Part model, mm, in its own coordinate system. A direction names the side the tool comes from. Coordinates: 2 decimals unless noted, no trailing zeros. Loops run counter-clockwise (first coordinate to the right, second up) from the corner with the lowest first, then second, coordinate; pieces in that order, holes last.
```python
from build123d import *

# Parameters (mm, degrees)
BOSS_EXTRUDE1_DEPTH     = 40
CUT_EXTRUDE1_DEPTH      = 2
CUT_EXTRUDE1_DEPTH_BACK = 34
SKETCH5_R               = 7.241016292
CUT_EXTRUDE2_DEPTH      = 19
SKETCH4_W               = 56.944481184
SKETCH4_H               = 24.913210518
SKETCH4_W_2             = 92.534781926
SKETCH4_H_2             = 83.281303733
CUT_EXTRUDE3_DEPTH      = 19
FILLET1_R               = 10
FILLET2_R               = 10
FILLET5_R               = 20
FILLET6_R               = 20
FILLET11_R              = 10
FILLET12_R              = 10


with BuildPart() as part:
    # Sketch1 → Boss-Extrude1 (new body)
    with BuildSketch(Plane.XY):
        Polygon((-15.339960816, 87.909775446), (15.339960816, 87.909775446), (96.75975284, 65.883165043), (99.51307914, 15.143294652), (65.29316655, -26.549932182), (65.29316655, -87.909775446), (-65.29316655, -87.909775446), (-65.29316655, -26.549932182), (-99.51307914, 15.143294652), (-96.75975284, 65.883165043), align=None)
    extrude(amount=BOSS_EXTRUDE1_DEPTH)

    # Sketch3 → Cut-Extrude1 (cut, two sides: drawn at the far end of the back side and taken through both)
    with BuildSketch(Plane.XY.offset(40).offset(-CUT_EXTRUDE1_DEPTH_BACK)):
        Polygon((-92.534781925, 62.816880807), (-16.371538341, 83.815158244), (15.303829318, 83.815158244), (92.673798797, 62.816880807), (95.770608339, 16.193586837), (62.268759659, -24.735259015), (62.268759659, -84.882867266), (60.147608251, -84.882867266), (-61.571220281, -84.882867266), (-61.571220281, -24.735259015), (-95.026102977, 16.193586837), align=None)
    extrude(amount=CUT_EXTRUDE1_DEPTH + CUT_EXTRUDE1_DEPTH_BACK, mode=Mode.SUBTRACT)

    # Sketch5 → Cut-Extrude2 (cut)
    with BuildSketch(Plane(origin=(0, 87.909775446, 0), x_dir=(1, 0, 0), z_dir=(0, 1, 0))):
        with Locations(Location((0, -19.844342197, 0), (0, 0, 270))):
            Circle(SKETCH5_R)
    extrude(amount=-CUT_EXTRUDE2_DEPTH, mode=Mode.SUBTRACT)

    # Sketch4 → Cut-Extrude3 (cut)
    with BuildSketch(Plane.XY.offset(6)):
        with Locations((0, 44.665827429)):
            Rectangle(SKETCH4_W, SKETCH4_H)
        with Locations((0, -35.05644623)):
            Rectangle(SKETCH4_W_2, SKETCH4_H_2)
    extrude(amount=-CUT_EXTRUDE3_DEPTH, mode=Mode.SUBTRACT)

    # Fillet1
    fillet1_edges = [part.edges().sort_by_distance(p)[0] for p in [
        (96.75975284, 65.883165043, 20),
    ]]
    fillet(fillet1_edges, radius=FILLET1_R)

    # Fillet2
    fillet2_edges = [part.edges().sort_by_distance(p)[0] for p in [
        (-96.75975284, 65.883165043, 20),
    ]]
    fillet(fillet2_edges, radius=FILLET2_R)

    # Fillet5
    fillet5_edges = [part.edges().sort_by_distance(p)[0] for p in [
        (-99.51307914, 15.143294652, 20),
    ]]
    fillet(fillet5_edges, radius=FILLET5_R)

    # Fillet6
    fillet6_edges = [part.edges().sort_by_distance(p)[0] for p in [
        (99.51307914, 15.143294652, 20),
    ]]
    fillet(fillet6_edges, radius=FILLET6_R)

    # Fillet11
    fillet11_edges = [part.edges().sort_by_distance(p)[0] for p in [
        (65.29316655, -87.909775446, 20),
    ]]
    fillet(fillet11_edges, radius=FILLET11_R)

    # Fillet12
    fillet12_edges = [part.edges().sort_by_distance(p)[0] for p in [
        (-65.29316655, -87.909775446, 20),
    ]]
    fillet(fillet12_edges, radius=FILLET12_R)


solid = part.part
```
Q1. Probe line 1 (X direction, y = -36, z = 9); line 2 (Y direction, x = 13.5, z = 6.5); line 3 (Y direction, x = -38.5, z = 27.5). List the from-to ranges inside material, lowest first.
Q2. Mould opens along Z. For faces 5 (the flat face through (0, 85, 40)), 6 (the flat face through (-93.798, 39.179, 22.762)), 7 (the cylindrical face through (-4.41, 85.89, 14.1)) say: released by +Z, released by -Z, zero draft, split by the parting line, or undercut.
Q3. Saw through at C-C (z = 30.5). List the corners of the cut face in (x, y).
Q4. Saw through at B-B (y = -55). List the corners of the cut face in (x, z).
Q5. Drop flat-ended pins along their axis: P1, Ø5, axis at y = -31.5, z = 3.5, coming from the -X side; P2, Ø2, axis at x = 27.5, z = 8, coming from the +Y side; P3, Ø16.5, axis at x = 0, z = 19.84, coming from the +Y side; P4, Ø5, axis at y = -41, z = 8.5, coming from the +X side. Give the stop position or say it passes through.
Q6. Saw through at A-A (x = 0). List the corners of the cut face in (y, z), plus the area to 3 significant figures.
Q7. Tool access for faces 1 (the flat face through (62.269, -54, 23)), 2 (the flat face through (65.293, -52, 20)), 3 (the flat face through (-65.293, -53, 20)), 4 (the flat face through (0, 57.122, 3)): list every direction of +Z, -Z, +X, -X, +Y, -Y with a clear straight run to the whole face (end or side of a thin tool).
Q8. Saw through at D-D (y = -18.5). List the corners of the cut face in (x, z).
Checked values:
1. line 1: x = -65.29 to -61.57, 62.27 to 65.29
1. line 2: y = -87.91 to -84.88, 83.82 to 87.91
1. line 3: y = -87.91 to -84.88, 77.71 to 81.64
2. face 5: released by +Z
2. face 6: zero draft
2. face 7: undercut
3. outline: (-99.09, 22.91) arc R20 ccw to (-94.58, 9.13) - (-65.29, -26.55) - (-65.29, -77.91) arc R10 ccw to (-55.29, -87.91) - (55.29, -87.91) arc R10 ccw to (65.29, -77.91) - (65.29, -26.55) - (94.58, 9.13) arc R20 ccw to (99.09, 22.91) - (97.15, 58.66) arc R10 ccw to (89.78, 67.77) - (15.34, 87.91) - (-15.34, 87.91) - (-89.78, 67.77) arc R10 ccw to (-97.15, 58.66) - close; hole (-95.03, 16.19) - (-61.57, -24.74) - (-61.57, -84.88) - (62.27, -84.88) - (62.27, -24.74) - (95.77, 16.19) - (92.67, 62.82) - (15.3, 83.82) - (-16.37, 83.82) - (-92.53, 62.82) - close
4. outline: (-65.29, 0) - (-46.27, 0) - (-46.27, 6) - (-61.57, 6) - (-61.57, 40) - (-65.29, 40) - close; (46.27, 0) - (65.29, 0) - (65.29, 40) - (62.27, 40) - (62.27, 6) - (46.27, 6) - close
5. P1: stops at x = -65.29
5. P2: stops at y = 84.89
5. P3: stops at y = 87.91
5. P4: stops at x = 65.29
6. outline: (-87.91, 0) - (-76.7, 0) - (-76.7, 6) - (-84.88, 6) - (-84.88, 40) - (-87.91, 40) - close; (6.58, 0) - (32.21, 0) - (32.21, 6) - (6.58, 6) - close; (57.12, 0) - (87.91, 0) - (87.91, 12.6) - (83.82, 12.6) - (83.82, 6) - (57.12, 6) - close; (83.82, 27.09) - (87.91, 27.09) - (87.91, 40) - (83.82, 40) - close
6. area: 589 mm2
7. face 1: +Z
7. face 2: +Z, -Z, +X, -Y
7. face 3: +Z, -Z, -X, -Y
7. face 4: +Z, -Z
8. outline: (-71.9, 0) - (-46.27, 0) - (-46.27, 6) - (-66.67, 6) - (-66.67, 40) - (-71.9, 40) - close; (46.27, 0) - (71.9, 0) - (71.9, 40) - (67.37, 40) - (67.37, 6) - (46.27, 6) - close
